```python
from build123d import *

# Parameters (mm, degrees)
F0_W     = 40
F0_H     = 40
F0_R     = 1.5
F0_R_2   = 13.5
F1_DEPTH = 2.5
F0_R_3   = 10.5
F2_DEPTH = 7.5
F3_SIZE  = 1
F4_SIZE  = 1
F5_SIZE  = 1


with BuildPart() as f1:
    # F0 (on Top) → F1 (new body)
    with BuildSketch(Plane.XY):
        Rectangle(F0_W, F0_H)
        with Locations((-16, -16)):
            Circle(F0_R, mode=Mode.SUBTRACT)
        with Locations((16, -16)):
            Circle(F0_R, mode=Mode.SUBTRACT)
        with Locations((-16, 16)):
            Circle(F0_R, mode=Mode.SUBTRACT)
        Circle(F0_R_2, mode=Mode.SUBTRACT)
        with Locations((16, 16)):
            Circle(F0_R, mode=Mode.SUBTRACT)
    extrude(amount=F1_DEPTH)

    # F0 (on Top) → F2 (join)
    with BuildSketch(Plane.XY):
        Circle(F0_R_2)
        Circle(F0_R_3, mode=Mode.SUBTRACT)
    extrude(amount=F2_DEPTH)

    # F3
    f3_edges = [f1.edges().sort_by_distance(p)[0] for p in [
        (-10.5, 0, 7.5),
    ]]
    chamfer(f3_edges, length=F3_SIZE)

    # F4
    f4_edges = [f1.edges().sort_by_distance(p)[0] for p in [
        (-17.5, -16, 2.5),
    ]]
    chamfer(f4_edges, length=F4_SIZE)

    # F5
    f5_edges = [f1.edges().sort_by_distance(p)[0] for p in [
        (17.5, -16, 1.25),
        (14.5, -16, 0),
        (14.5, -16, 2.5),
        (17.5, 16, 1.25),
        (14.5, 16, 0),
        (14.5, 16, 2.5),
        (-17.5, 16, 2.5),
    ]]
    chamfer(f5_edges, length=F5_SIZE)


solid = f1.part
```
CAD build for the part. Positions are in the model's coordinates, mm. A direction names the side the tool comes from. Coordinates: 2 decimals unless noted, no trailing zeros. Order: outer loops, then holes, each group sorted by start corner. A loop starts at its lowest first (then second) coordinate and runs counter-clockwise, first axis right, second up. Notation, with made-up numbers: (12, 64) - (23, 64) arc R21 cw to (23, 71) - close; hole circle Ø3 at (69.5, 46.25). An arc over 180 degrees is marked (long way). Use a Markdown table: item, result. Add a question column.
(1) Which spindle directions (+Z, -Z, +X, -X, +Y, -Y) get a long thin tool onto all of the face, cutting with end or side? Do faces 1 (the face through (0, 14, 2.5)), 2 (the face through (-17.5, -15.93, 0.74)). Say none if no direction does.
(2) Saw through at B-B (x = 16). Give the cut face in (y, z).
(3) Pull direction Y, two halves, no side cores. Call faces 3 (the face through (14.5, -15.93, 1.25)), 4 (the face through (-20, 0, 1)), 5 (the face through (0, 20, 1)): +Y half, -Y half, draft (parallel to the pull), parting line (faces both ways), or undercut.
(4) Flat gauge pins, fed straight in: pin 1 (3.5 mm diameter, centred on x = 16, y = -16, fed in from -Z); pin 2 (4 mm diameter, centred on x = 15.5, y = 13, fed in from +Z); pin 3 (3.5 mm diameter, centred on x = -16, y = 16, fed in from +Z). Where does each tip first touch, or does it go through?
(5) Saw through at A-A (y = 0). Give the cut face in (x, z).
(6) Saw through at C-C (y = 16). Give the cut face in (x, z).
(7) Drill centre lines: line 1 along Y through (x, z) = (16, 1.4); line 2 along Z through (x, y) = (14, 2.5); line 3 along Y through (x, z) = (8.5, 6). Where is each one in solid material? Low to high. Write a range as [from, to].
Solved:
| question | item | result |
|---|---|---|
| 1 | face 1 | +Z |
| 1 | face 2 | +Z, -Z |
| 2 | outline | (-20, 0) - (-18.5, 0) - (-17.5, 1) - (-17.5, 1.5) - (-18.5, 2.5) - (-20, 2.5) - close; (-14.5, 1) - (-13.5, 0) - (13.5, 0) - (14.5, 1) - (14.5, 1.5) - (13.5, 2.5) - (-13.5, 2.5) - (-14.5, 1.5) - close; (17.5, 1) - (18.5, 0) - (20, 0) - (20, 2.5) - (18.5, 2.5) - (17.5, 1.5) - close |
| 3 | face 3 | undercut |
| 3 | face 4 | draft |
| 3 | face 5 | +Y half |
| 4 | pin 1 | stops at z = 0.75 |
| 4 | pin 2 | stops at z = 2.5 |
| 4 | pin 3 | stops at z = 1.75 |
| 5 | outline | (-20, 0) - (-10.5, 0) - (-10.5, 6.5) - (-11.5, 7.5) - (-13.5, 7.5) - (-13.5, 2.5) - (-20, 2.5) - close; (10.5, 0) - (20, 0) - (20, 2.5) - (13.5, 2.5) - (13.5, 7.5) - (11.5, 7.5) - (10.5, 6.5) - close |
| 6 | outline | (-20, 0) - (-17.5, 0) - (-17.5, 1.5) - (-18.5, 2.5) - (-20, 2.5) - close; (-14.5, 0) - (13.5, 0) - (14.5, 1) - (14.5, 1.5) - (13.5, 2.5) - (-13.5, 2.5) - (-14.5, 1.5) - close; (17.5, 1) - (18.5, 0) - (20, 0) - (20, 2.5) - (18.5, 2.5) - (17.5, 1.5) - close |
| 7 | line 1 | y = [-20, -17.5], [-14.5, 14.5], [17.5, 20] |
| 7 | line 2 | z = [0, 2.5] |
| 7 | line 3 | y = [-10.49, -6.16], [6.16, 10.49] |
